Autodesk Fusion 360 part; units mm, degrees
sketch "Sketch1" plane through (0, 0, 0) normal (0, 0, 1) x (1, 0, 0)
  line L0 (10.5, 10.5) -> (-10.5, 10.5)
  line L1 (-10.5, 10.5) -> (-10.5, -10.5)
  line L2 (-10.5, -10.5) -> (10.5, -10.5)
  line L3 (10.5, -10.5) -> (10.5, 10.5)
  line L4 (10.5, 10.5) -> (-10.5, -10.5) construction
  line L5 (-10.5, 10.5) -> (10.5, -10.5) construction
  line L6 (7.5, 7.5) -> (-7.5, 7.5)
  line L7 (-7.5, 7.5) -> (-7.5, -7.5)
  line L8 (-7.5, -7.5) -> (7.5, -7.5)
  line L9 (7.5, -7.5) -> (7.5, 7.5)
  line L10 (7.5, 7.5) -> (-7.5, -7.5) construction
  line L11 (-7.5, 7.5) -> (7.5, -7.5) construction
  line L12 (10.5, 10.5) -> (27.7245, 2.7349)
  line L13 (27.7245, -2.7349) -> (10.5, -10.5)
  line L14 (-10.5, 10.5) -> (-27.7245, 2.7349)
  line L15 (-27.7245, -2.7349) -> (-10.5, -10.5)
  arc A0 (27.7245, -2.7349) -> (27.7245, 2.7349) centre (26.4916, 0) ccw
  arc A1 (-27.7245, 2.7349) -> (-27.7245, -2.7349) centre (-26.4916, 0) ccw
  line L16 (26.4916, 0) -> (0, 0) construction
  line L17 (0, 0) -> (-26.4916, 0) construction
  line L18 (7.5, 7.5) -> (10.5, 7.5) construction
  line L19 (7.5, -7.5) -> (10.5, -7.5) construction
  line L20 (-7.5, -7.5) -> (-10.5, -7.5) construction
  line L21 (-7.5, 7.5) -> (-10.5, 7.5) construction
  line L22 (10.5, 7.5) -> (27.1365, 0)
  line L23 (10.5, -7.5) -> (27.1365, 0)
  line L24 (-10.5, 7.5) -> (-27.1365, 0)
  line L25 (-10.5, -7.5) -> (-27.1365, 0)
  line L26 (-24.3008, 1.2784) -> (-24.3008, -1.2784)
  line L27 (24.3008, -1.2784) -> (24.3008, 1.2784)
  dimension "d1" = 15
  dimension "d2" = 3
  dimension "d3" = 3
  dimension "d4" = 3
extrude "Extrude1" add sketch "Sketch1" along normal blind 15 contours L0 L1 L2 L3 | L3 L12 L13 A0 L22 L23 | L1 L14 L15 A1 L24 L25 | L22 L23 L27 | L24 L25 L26
fillet "Fillet1" radius 5 4 edges at (-10.5, -10.5, 7.5) (10.5, -10.5, 7.5) (10.5, 10.5, 7.5) (-10.5, 10.5, 7.5)
fillet "Fillet2" radius 2 8 edges at (-10.5, 7.5, 7.5) (-10.5, -7.5, 7.5) (-24.3008, -1.2784, 7.5) (-24.3008, 1.2784, 7.5) (10.5, 7.5, 7.5) (10.5, -7.5, 7.5) (24.3008, -1.2784, 7.5) (24.3008, 1.2784, 7.5)
sketch "Sketch2" plane through (0, 10.5, 0) normal (0, 1, 0) x (-1, 0, 0)
  line L0 (9.4251, 0) -> (9.4251, 15)
  line L1 (9.4251, 15) -> (-9.4251, 15)
  line L2 (-9.4251, 15) -> (-9.4251, 0)
  line L3 (-9.4251, 0) -> (9.4251, 0)
  circle A0 centre (0, 7.5) radius 1.65
  dimension "d13" = 3.3
extrude "Extrude2" cut sketch "Sketch2" against normal blind 35 contours A0
chamfer "Chamfer1" distance 0.5 angle 45 2 faces at (2.5, -9.5, 0) (2.5, -9.5, 15)
Geometry check sheet. Reference: the model listing, model coordinates, mm. A direction names the side the tool comes from. Coordinates: 2 decimals unless noted, no trailing zeros. Loops run counter-clockwise (first coordinate to the right, second up) from the corner with the lowest first, then second, coordinate; pieces in that order, holes last.
Item 1: Sectioned sample at C-C, the plane x = 21. Record the boundary of the cut face in (y, z).
Item 2: Thickness scan on line 1 (Z direction, x = 0, y = 9.55); line 2 (Y direction, x = 5.5, z = 10.25); line 3 (X direction, y = -5.5, z = 13.25). Record the ranges inside material, lowest first.
Item 3: Sectioned sample at B-B, the plane z = 7.5. Count the separate pieces of the cut face and the enclosed holes in it, then the cut area to 3 significant figures.
Item 4: Release check for a two-part mould opening along X. For faces 1 (the face through (-29.13, 0.04, 0.14)), 2 (the face through (-18.24, -4.281, 0.253)), 3 (the face through (-2.3, 8.2, 15)), 4 (the face through (-11.39, 6.07, 7.6)) record: released by +X, released by -X, zero draft, split by the parting line, or undercut.
Item 5: Go/stop test with flat-tipped pins: pin 1 Ø6 at (x, z) = (21, 12.5) entering from +Y; pin 2 Ø1 at (y, z) = (8, 7.5) entering from -X. Record where each tip stops, or that it passes through.
Item 6: Sectioned sample at A-A, the plane x = 0. Record the boundary of the cut face in (y, z), then the cut area to 3 significant figures.
Item 7: Access from +Z, -Z, +X, -X, +Y, -Y to the whole of each face (thin tool, end or side, straight path). Record for faces 5 (the face through (-18.38, 4.226, 14.753)), 6 (the face through (7.5, 0, 7)), 7 (the face through (11.363, -6.22, 0.358)), 8 (the face through (19.61, -6.12, 0.25)).
Check result:
1. outline: (-5.77, 0.5) - (-5.22, 0) - (-3.31, 0) - (-2.77, 0.5) - (-2.77, 14.5) - (-3.31, 15) - (-5.22, 15) - (-5.77, 14.5) - close; (2.77, 0.5) - (3.31, 0) - (5.22, 0) - (5.77, 0.5) - (5.77, 14.5) - (5.22, 15) - (3.31, 15) - (2.77, 14.5) - close
2. line 1: z = 0 to 5.85, 9.15 to 15
2. line 2: y = -10.5 to -7.5, 7.5 to 10.5
2. line 3: x = -21.59 to -14.94, -10.83 to -7.5, 7.5 to 10.83, 14.94 to 21.59
3. separate pieces: 2
3. enclosed holes: 2
3. area: 434 mm2
4. face 1: released by -X
4. face 2: undercut
4. face 3: zero draft
4. face 4: undercut
5. pin 1: stops at y = 7.12
5. pin 2: stops at x = -17.15
6. outline: (-10.5, 0.5) - (-10, 0) - (-8, 0) - (-7.5, 0.5) - (-7.5, 5.85) - (-10.5, 5.85) - close; (-10.5, 9.15) - (-7.5, 9.15) - (-7.5, 14.5) - (-8, 15) - (-10, 15) - (-10.5, 14.5) - close; (7.5, 0.5) - (8, 0) - (10, 0) - (10.5, 0.5) - (10.5, 5.85) - (7.5, 5.85) - close; (7.5, 9.15) - (10.5, 9.15) - (10.5, 14.5) - (10, 15) - (8, 15) - (7.5, 14.5) - close
6. area: 69.2 mm2
7. face 5: +Z
7. face 6: +Z, -Z
7. face 7: -Z
7. face 8: -Z, +X, -Y
